For this review, take the finished solid that the model builds, in its own axes (mm). Round coordinates to 2 decimals unless told otherwise and drop trailing zeros. Order: outer loops, then holes, each group sorted by start corner. A loop starts at its lowest first (then second) coordinate and runs counter-clockwise, first axis right, second up. Notation, with made-up numbers: M 23,75 L 73,75 A12 cw 73,97 Z; hole C -31,25 d6. An arc over 180 degrees is marked long. Answer as a JSON object with one key per item and string values.
from build123d import *

# Parameters (mm, degrees)
SKETCH1_W                      = 32
SKETCH1_H                      = 51
SKETCH1_R                      = 2.25
BOSS_EXTRUDE1_DEPTH            = 4
SKETCH1_3_R                    = 2.25
BOSS_EXTRUDE2_DEPTH            = 2
F_2_5MM_DOWEL_HOLE1_AT_2_COUNT = 2
F_2_5MM_DOWEL_HOLE1_AT_2_PITCH = 11
F_2_5MM_DOWEL_HOLE1_AT_3_COUNT = 2
F_2_5MM_DOWEL_HOLE1_AT_3_PITCH = 21.09502311
F_2_5MM_DOWEL_HOLE1_AT_4_COUNT = 2
F_2_5MM_DOWEL_HOLE1_AT_4_PITCH = 18
M4_CLEARANCE_HOLE1_AT_2_COUNT  = 2
M4_CLEARANCE_HOLE1_AT_2_PITCH  = 20
FILLET1_R                      = 1
CHAMFER1_SIZE                  = 1
CHAMFER2_SIZE                  = 0.1


with BuildPart() as part:
    # Sketch1 → Boss-Extrude1 (new body)
    with BuildSketch(Plane.XY):
        with Locations((0, -15)):
            Rectangle(SKETCH1_W, SKETCH1_H)
        with Locations((9, 5.5)):
            Circle(SKETCH1_R, mode=Mode.SUBTRACT)
        with Locations((9, -5.5)):
            Circle(SKETCH1_R, mode=Mode.SUBTRACT)
        with Locations((-9, -5.5)):
            Circle(SKETCH1_R, mode=Mode.SUBTRACT)
        with Locations((-9, 5.5)):
            Circle(SKETCH1_R, mode=Mode.SUBTRACT)
        with Locations((-9, 5.5)):
            Circle(SKETCH1_R)
        with Locations((9, 5.5)):
            Circle(SKETCH1_R)
        with Locations((-9, -5.5)):
            Circle(SKETCH1_R)
        with Locations((9, -5.5)):
            Circle(SKETCH1_R)
    extrude(amount=BOSS_EXTRUDE1_DEPTH)

    # Sketch1_3 → Boss-Extrude2 (add)
    with BuildSketch(Plane.XY):
        with Locations((-9, 5.5)):
            Circle(SKETCH1_3_R)
        with Locations((9, 5.5)):
            Circle(SKETCH1_3_R)
        with Locations((-9, -5.5)):
            Circle(SKETCH1_3_R)
        with Locations((9, -5.5)):
            Circle(SKETCH1_3_R)
    extrude(amount=-BOSS_EXTRUDE2_DEPTH)

    # Sketch5 → 2.5mm Dowel Hole1 (revolve, cut)
    with BuildSketch(Plane(origin=(-9, 5.5, -2), x_dir=(0, 1, 0), z_dir=(1, 0, 0))):
        Polygon((0, 0), (0, 6), (1.5, 6), (1.25, 5.75), (1.25, 0.25), (1.5, 0), align=None)
    f_2_5mm_dowel_hole1 = revolve(axis=Axis((-9, 5.5, -8.35), (0, 0, 1)), mode=Mode.SUBTRACT)

    # 2.5mm Dowel Hole1 at 2: 2.5mm Dowel Hole1 ×2
    with Locations(*[(0, -i * F_2_5MM_DOWEL_HOLE1_AT_2_PITCH, 0) for i in range(1, F_2_5MM_DOWEL_HOLE1_AT_2_COUNT)]):
        add(f_2_5mm_dowel_hole1, mode=Mode.SUBTRACT)

    # 2.5mm Dowel Hole1 at 3: 2.5mm Dowel Hole1 ×2
    with Locations(*[Vector(0.853281834, -0.521450009, 0) * (i * F_2_5MM_DOWEL_HOLE1_AT_3_PITCH) for i in range(1, F_2_5MM_DOWEL_HOLE1_AT_3_COUNT)]):
        add(f_2_5mm_dowel_hole1, mode=Mode.SUBTRACT)

    # 2.5mm Dowel Hole1 at 4: 2.5mm Dowel Hole1 ×2
    with Locations(*[(i * F_2_5MM_DOWEL_HOLE1_AT_4_PITCH, 0, 0) for i in range(1, F_2_5MM_DOWEL_HOLE1_AT_4_COUNT)]):
        add(f_2_5mm_dowel_hole1, mode=Mode.SUBTRACT)

    # Sketch8 → M4 Clearance Hole1 (revolve, cut)
    with BuildSketch(Plane(origin=(-10, -34.5, 0), x_dir=(0, 1, 0), z_dir=(1, 0, 0))):
        Polygon((0, 0), (0, 4), (2.5, 4), (2.25, 3.75), (2.25, 0.25), (2.5, 0), align=None)
    m4_clearance_hole1 = revolve(axis=Axis((-10, -34.5, -6.35), (0, 0, 1)), mode=Mode.SUBTRACT)

    # M4 Clearance Hole1 at 2: M4 Clearance Hole1 ×2
    with Locations(*[(i * M4_CLEARANCE_HOLE1_AT_2_PITCH, 0, 0) for i in range(1, M4_CLEARANCE_HOLE1_AT_2_COUNT)]):
        add(m4_clearance_hole1, mode=Mode.SUBTRACT)

    # Fillet1
    fillet1_edges = [part.edges().sort_by_distance(p)[0] for p in [
        (-16, -40.5, 2),
        (-16, 10.5, 2),
        (16, 10.5, 2),
        (16, -40.5, 2),
    ]]
    fillet(fillet1_edges, radius=FILLET1_R)

    # Chamfer1
    chamfer1_edges = [part.edges().sort_by_distance(p)[0] for p in [
        (0, 10.5, 0),
        (0, 10.5, 4),
        (0, -40.5, 0),
        (-16, -15, 0),
        (16, -15, 0),
        (-15.707106781, 10.207106781, 0),
        (-15.707106781, -40.207106781, 0),
        (15.707106781, -40.207106781, 0),
        (15.707106781, 10.207106781, 0),
        (16, -15, 4),
        (0, -40.5, 4),
        (-16, -15, 4),
        (-15.707106781, 10.207106781, 4),
        (-15.707106781, -40.207106781, 4),
        (15.707106781, -40.207106781, 4),
        (15.707106781, 10.207106781, 4),
    ]]
    chamfer(chamfer1_edges, length=CHAMFER1_SIZE)

    # Chamfer2
    chamfer2_edges = [part.edges().sort_by_distance(p)[0] for p in [
        (-11.25, 5.5, -2),
        (-11.25, 5.5, 0),
        (6.75, 5.5, -2),
        (6.75, 5.5, 0),
        (-11.25, -5.5, -2),
        (-11.25, -5.5, 0),
        (6.75, -5.5, -2),
        (6.75, -5.5, 0),
    ]]
    chamfer(chamfer2_edges, length=CHAMFER2_SIZE)


solid = part.part
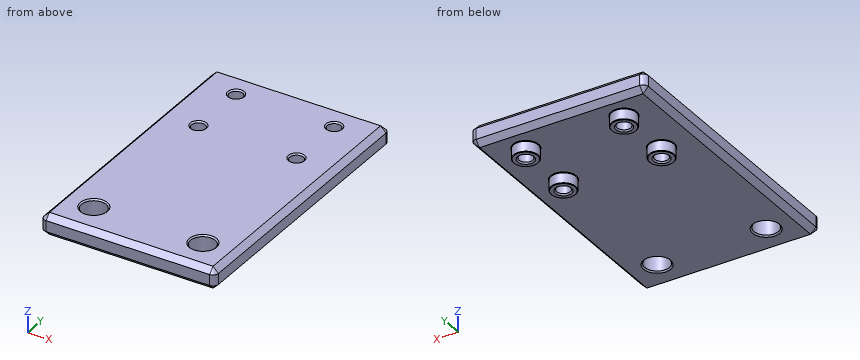
1) Add section A-A on z = -0.75. State the section outline as (x, y) points.
Geometry check:
{"outline": "C -9,-5.5 d4.5; C -9,5.5 d4.5; C 9,-5.5 d4.5; C 9,5.5 d4.5; hole C -9,-5.5 d2.5; hole C -9,5.5 d2.5; hole C 9,-5.5 d2.5; hole C 9,5.5 d2.5"}
2) For L1, parallel to X at y = -5.5, z = 1.5; L2, parallel to X at y = -34.5, z = 1.65; L3, parallel to Y at x = -10, z = 2.1, list the stretches that pass through material, from the lowest coordinate up.
Geometry check:
{"L1": "x = -16 to -10.25, -7.75 to 7.75, 10.25 to 16", "L2": "x = -16 to -12.25, -7.75 to 7.75, 12.25 to 16", "L3": "y = -40.5 to -36.75, -32.25 to -6.25, -4.75 to 4.75, 6.25 to 10.5"}
3) Insertion check: P1, Ø10, axis at x = 2, y = -17, coming from the -Z side. The pin has a flat end and moves straight along its axis. Give the tip position at first contact, or say it passes through.
Geometry check:
{"P1": "stops at z = 0"}
4) Add section C-C on x = 5.5. State the section outline as (y, z) points, and give its area (3 significant figures).
Geometry check:
{"outline": "M -40.5,1 L -39.5,0 L 9.5,0 L 10.5,1 L 10.5,3 L 9.5,4 L -39.5,4 L -40.5,3 Z", "area": "202 mm²"}
5) Add section B-B on y = -34.5. State the section outline as (x, z) points, and give its area (4 significant figures).
Geometry check:
{"outline": "M -16,1 L -15,0 L -12.5,0 L -12.25,0.25 L -12.25,3.75 L -12.5,4 L -15,4 L -16,3 Z; M -7.75,0.25 L -7.5,0 L 7.5,0 L 7.75,0.25 L 7.75,3.75 L 7.5,4 L -7.5,4 L -7.75,3.75 Z; M 12.25,0.25 L 12.5,0 L 15,0 L 16,1 L 16,3 L 15,4 L 12.5,4 L 12.25,3.75 Z", "area": "89.75 mm²"}
6) Add section D-D on z = 2.25. State the section outline as (x, y) points, and give its area (3 significant figures).
Geometry check:
{"outline": "M -16,-39.5 A1 ccw -15,-40.5 L 15,-40.5 A1 ccw 16,-39.5 L 16,9.5 A1 ccw 15,10.5 L -15,10.5 A1 ccw -16,9.5 Z; hole C -10,-34.5 d4.5; hole C -9,-5.5 d2.5; hole C -9,5.5 d2.5; hole C 10,-34.5 d4.5; hole C 9,-5.5 d2.5; hole C 9,5.5 d2.5", "area": "1,580 mm²"}
